from build123d import *

# Parameters (mm, degrees)
F0_R     = 11
F1_DEPTH = 7
F2_R     = 2


with BuildPart() as f1:
    # F0 (on Top) → F1 (new body)
    with BuildSketch(Plane.XY):
        with BuildLine():
            ThreePointArc((21.566864, 19.5), (0, 28), (-21.566864, 19.5))
            Line((-21.566864, 19.5), (-21.566864, -19.5))
            ThreePointArc((-21.566864, -19.5), (0, -28), (21.566864, -19.5))
            Line((21.566864, -19.5), (21.566864, 19.5))
        make_face()
        with BuildLine():
            ThreePointArc((-8.37799, -17.349157), (-18.3602, -12.98084), (-7.566864, -14.474359))
            ThreePointArc((-7.566864, -14.474359), (-7.590208, -14.980559), (-7.660042, -15.482462))
            Line((-7.660042, -15.482462), (-4.688874, -16.625202))
            ThreePointArc((-4.688874, -16.625202), (0.502097, -14.022966), (5.133411, -17.525641))
            Line((5.133411, -17.525641), (7.933453, -16.448718))
            ThreePointArc((7.933453, -16.448718), (12.062812, -9.066783), (18.566864, -14.474359))
            ThreePointArc((18.566864, -14.474359), (15.05405, -19.602818), (9.00283, -18.18025))
            Line((9.00283, -18.18025), (5.5, -19.5))
            ThreePointArc((5.5, -19.5), (-0.5062, -24.976656), (-5.406822, -18.491897))
            Line((-5.406822, -18.491897), (-8.37799, -17.349157))
        make_face(mode=Mode.SUBTRACT)
        Circle(F0_R, mode=Mode.SUBTRACT)
        with BuildLine():
            ThreePointArc((8.37799, 17.349157), (14.560382, 19.767695), (18.566864, 14.474359))
            ThreePointArc((18.566864, 14.474359), (12.560664, 8.997703), (7.660042, 15.482462))
            Line((7.660042, 15.482462), (4.688874, 16.625202))
            ThreePointArc((4.688874, 16.625202), (0, 14), (-4.688874, 16.625202))
            Line((-4.688874, 16.625202), (-7.660042, 15.482462))
            ThreePointArc((-7.660042, 15.482462), (-7.590208, 14.980559), (-7.566864, 14.474359))
            ThreePointArc((-7.566864, 14.474359), (-18.3602, 12.98084), (-8.37799, 17.349157))
            Line((-8.37799, 17.349157), (-5.406822, 18.491897))
            ThreePointArc((-5.406822, 18.491897), (-0.5062, 24.976656), (5.5, 19.5))
            ThreePointArc((5.5, 19.5), (5.476656, 18.9938), (5.406822, 18.491897))
            Line((5.406822, 18.491897), (8.37799, 17.349157))
        make_face(mode=Mode.SUBTRACT)
    extrude(amount=F1_DEPTH)

    # F2
    f2_edges = [f1.edges().sort_by_distance(p)[0] for p in [
        (21.566864, 19.5, 3.5),
        (-21.566864, 19.5, 3.5),
        (0, 28, 0),
        (0, 28, 7),
        (-21.566864, -19.5, 3.5),
        (-21.566864, 0, 0),
        (-21.566864, 0, 7),
        (21.566864, -19.5, 3.5),
        (0, -28, 0),
        (0, -28, 7),
        (21.566864, 0, 0),
        (21.566864, 0, 7),
    ]]
    fillet(f2_edges, radius=F2_R)


solid = f1.part
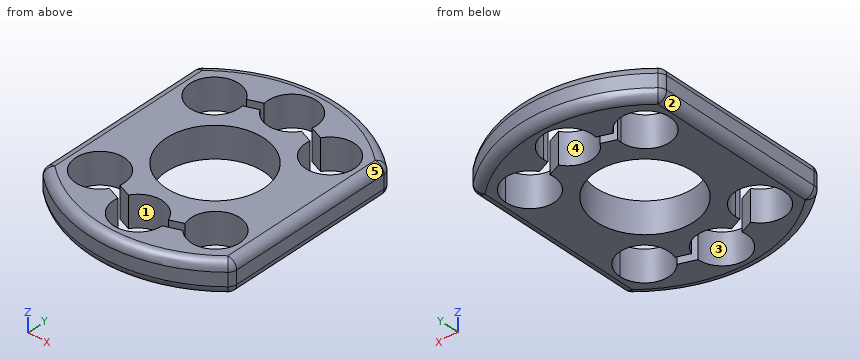
Can you work these out from the model? Positions are in its coordinate system, mm. Face numbers are marked on the shaded views. A direction names the side the tool comes from. Coordinates: 2 decimals unless noted, no trailing zeros. Order: outer loops, then holes, each group sorted by start corner. A loop starts at its lowest first (then second) coordinate and runs counter-clockwise, first axis right, second up. Notation, with made-up numbers: (-29, -13.75) -> (-25, -13.75) arc R32 ccw to (-25, 16.25) -> close; hole circle Ø2 at (-34, -17). An arc over 180 degrees is marked (long way). Use one line per item in the form item = value.
Q1. Which directions (+Z, -Z, +X, -X, +Y, -Y) give clear straight access to the entire face, cutting with the end or side of a thin tool? Please do the marked faces 4 and 5.
From the geometry:
face_4 = +Z, -Z
face_5 = +Z, +X, +Y, -Y
Q2. Imagine slicing it at B-B, the plane z = 3.5. List the corners of the cut face in (x, y) for me, then the cut area to 3 significant figures.
From the geometry:
outline = (-21.57, -18.61) arc R2 ccw to (-20.89, -20.11) arc R31.61 ccw to (20.89, -20.11) arc R2 ccw to (21.57, -18.61) -> (21.57, 18.61) arc R2 ccw to (20.89, 20.11) arc R31.61 ccw to (-20.89, 20.11) arc R2 ccw to (-21.57, 18.61) -> close; hole circle Ø22 at (0, 0); hole (-8.38, -17.35) -> (-5.41, -18.49) arc R5.5 ccw (long way) to (5.5, -19.5) -> (9, -18.18) arc R5.5 ccw (long way) to (7.93, -16.45) -> (5.13, -17.53) arc R5.5 ccw to (-4.69, -16.63) -> (-7.66, -15.48) arc R5.5 ccw to (-7.57, -14.47) arc R5.5 ccw (long way) to start; hole (-8.38, 17.35) arc R5.5 ccw (long way) to (-7.57, 14.47) arc R5.5 ccw to (-7.66, 15.48) -> (-4.69, 16.63) arc R5.5 ccw to (4.69, 16.63) -> (7.66, 15.48) arc R5.5 ccw (long way) to (8.38, 17.35) -> (5.41, 18.49) arc R5.5 ccw to (5.5, 19.5) arc R5.5 ccw (long way) to (-5.41, 18.49) -> close
area = 1,210 mm²
Q3. Imagine slicing it at C-C, the plane x = 0. List the corners of the cut face in (y, z) for me, then the cut area to 3 significant figures.
From the geometry:
outline = (-28, 2) arc R2 ccw to (-26, 0) -> (-25, 0) -> (-25, 7) -> (-26, 7) arc R2 ccw to (-28, 5) -> close; (-14, 0) -> (-11, 0) -> (-11, 7) -> (-14, 7) -> close; (11, 0) -> (14, 0) -> (14, 7) -> (11, 7) -> close; (25, 0) -> (26, 0) arc R2 ccw to (28, 2) -> (28, 5) arc R2 ccw to (26, 7) -> (25, 7) -> close
area = 80.6 mm²
Q4. Imagine slicing it at A-A, the plane y = 0. List the corners of the cut face in (x, z) for me.
From the geometry:
outline = (-21.57, 2) arc R2 ccw to (-19.57, 0) -> (-11, 0) -> (-11, 7) -> (-19.57, 7) arc R2 ccw to (-21.57, 5) -> close; (11, 0) -> (19.57, 0) arc R2 ccw to (21.57, 2) -> (21.57, 5) arc R2 ccw to (19.57, 7) -> (11, 7) -> close
Q5. We'd pull the mould along Y, two halves only. Please class the marked faces 1, 2 and 3: released by +Y, released by -Y, zero draft, split by the parting line, or undercut.
From the geometry:
face_1 = undercut
face_2 = zero draft
face_3 = undercut
Q6. Will this pin go through, and if not, where does the flat tip stop? P1, Ø9, axis at x = 13.07, y = -14.47, coming from the +Z side.
From the geometry:
P1 = through
Q7. I need wall thicknesses on L1, parallel to X at y = 13.5, z = 4; L2, parallel to Y at x = 6, z = 2; L3, parallel to X at y = 19.5, z = 3.5. Which ranges of each line are inside material? Lowest first, please.
From the geometry:
L1 = -21.57 to -18.48, -7.65 to 7.65, 18.48 to 21.57
L2 = -27.43 to -19.31, -17.19 to -9.22, 9.22 to 16.12, 18.26 to 27.43
L3 = -21.36 to -15.3, -10.83 to -5.5, 5.5 to 10.83, 15.3 to 21.36
Q8. Imagine slicing it at D-D, the plane y = 12.5. List the corners of the cut face in (x, z) for me, then the cut area to 3 significant figures.
From the geometry:
outline = (-21.57, 2) arc R2 ccw to (-19.57, 0) -> (-18.2, 0) -> (-18.2, 7) -> (-19.57, 7) arc R2 ccw to (-21.57, 5) -> close; (-7.93, 0) -> (7.93, 0) -> (7.93, 7) -> (-7.93, 7) -> close; (18.2, 0) -> (19.57, 0) arc R2 ccw to (21.57, 2) -> (21.57, 5) arc R2 ccw to (19.57, 7) -> (18.2, 7) -> close
area = 155 mm²
